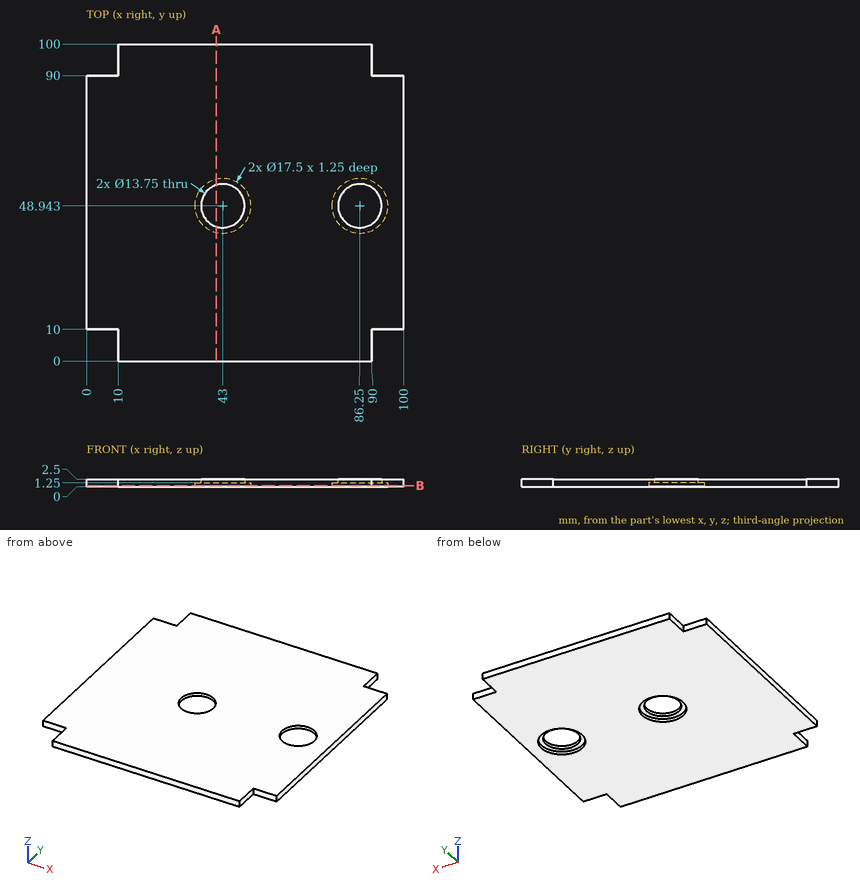
Answer from the drawing. Dimensions are ordinates in mm from the lowest x, y and z of the part. Give positions to 0.01 mm unless a question says otherwise; leave off trailing zeros. Order: outer loops, then holes, each group sorted by start corner. A loop starts at its lowest first (then second) coordinate and runs counter-clockwise, first axis right, second up. Notation, with made-up numbers: (-15, 74) - (42, 74) arc R31 ccw to (42, 100) - close; hole circle Ø6 at (16.25, 82). An arc over 180 degrees is marked (long way). One line per item, written item: value. Start each with the question number.
1) A cutting plane is placed at A-A on x = 41. Give the vertices of the cut face in (y, z), then the cut area to 3 significant figures.
2) Given pin 1 Ø0.8 at (y, z) = (4.5, 0.5) entering from -X; pin 2 Ø1.2 at (y, z) = (93.5, 1.5) entering from +X; pin 3 Ø0.8 at (x, z) = (4.5, 1.5) entering from -Y, each flat-ended and moving along its own axis, determine where each tip first touches the part or whether it passes through.
3) A cutting plane is placed at B-B on z = 0.4. Give the vertices of the cut face in (x, y), then the cut area to 3 significant figures.
4) Find the intervals of material crossed by L1, parallel to X at y = 47.5, z = 2.4; L2, parallel to X at y = 47, z = 2.05; L3, parallel to Y at x = 42.5, z = 1.7, in increasing order.
Answer sheet:
1. outline: (0, 0) - (40.42, 0) - (40.42, 1.25) - (42.37, 1.25) - (42.37, 2.5) - (0, 2.5) - close; (55.52, 1.25) - (57.46, 1.25) - (57.46, 0) - (100, 0) - (100, 2.5) - (55.52, 2.5) - close
1. area: 212 mm2
2. pin 1: stops at x = 10
2. pin 2: stops at x = 90
2. pin 3: stops at y = 10
3. outline: (0, 10) - (10, 10) - (10, 0) - (90, 0) - (90, 10) - (100, 10) - (100, 90) - (90, 90) - (90, 100) - (10, 100) - (10, 90) - (0, 90) - close; hole circle Ø17.5 at (43, 48.94); hole circle Ø17.5 at (86.25, 48.94)
3. area: 9,120 mm2
4. L1: x = 0 to 36.28, 49.72 to 79.53, 92.97 to 100
4. L2: x = 0 to 36.41, 49.59 to 79.66, 92.84 to 100
4. L3: y = 0 to 42.09, 55.8 to 100
